```python
from build123d import *

# Parameters (mm, degrees)
BOSS_EXTRUDE1_DEPTH = 3.175
SKETCH2_R           = 1.5875
CUT_EXTRUDE1_DEPTH  = 3.175
BOSS_EXTRUDE2_DEPTH = 3.175
CUT_EXTRUDE2_DEPTH  = 3.175
SKETCH5_W           = 1.5875
SKETCH5_H           = 12.7
CUT_EXTRUDE3_DEPTH  = 10.16
LPATTERN1_COUNT     = 2
LPATTERN1_PITCH     = 25.4
SKETCH9_R           = 1.5875
CUT_EXTRUDE7_DEPTH  = 7.62
SKETCH10_R          = 6.35
CUT_EXTRUDE8_DEPTH  = 5.08


with BuildPart() as part:
    # Sketch1 → Boss-Extrude1 (new body)
    with BuildSketch(Plane.XY):
        Polygon((0, 0), (-177.8, 0), (-232.7656, 382.27), (-80.3656, 382.27), align=None)
    extrude(amount=BOSS_EXTRUDE1_DEPTH)

    # Sketch2 → Cut-Extrude1 (cut)
    with BuildSketch(Plane.XY.offset(3.175)):
        with Locations((-127, 127)):
            Circle(SKETCH2_R)
        with Locations((-127, 299.72)):
            Circle(SKETCH2_R)
    extrude(amount=-CUT_EXTRUDE1_DEPTH, mode=Mode.SUBTRACT)

    # Sketch3 → Boss-Extrude2 (add)
    with BuildSketch(Plane.XY.offset(3.175)):
        Polygon((-63.5, 82.55), (63.5, 104.94352655), (63.5, 181.14352655), (-63.5, 181.14352655), align=None)
    extrude(amount=-BOSS_EXTRUDE2_DEPTH)

    # Sketch4 → Cut-Extrude2 (cut)
    with BuildSketch(Plane.XY.offset(3.175)):
        Polygon((-57.15, 104.14), (-44.642941537, 106.345331856), (-45.194274501, 109.472096472), (-57.701332964, 107.266764616), align=None)
        Polygon((-19.62882461, 110.755995569), (-7.121766147, 112.961327425), (-7.673099111, 116.088092041), (-20.180157574, 113.882760185), align=None)
    extrude(amount=-CUT_EXTRUDE2_DEPTH, mode=Mode.SUBTRACT)

    # Sketch5 → Cut-Extrude3 (cut)
    with BuildSketch(Plane.XY.offset(3.175)):
        with Locations((-126.20625, 203.2)):
            Rectangle(SKETCH5_W, SKETCH5_H)
        with Locations((-127.79375, 203.2)):
            Rectangle(SKETCH5_W, SKETCH5_H)
    cut_extrude3 = extrude(amount=-CUT_EXTRUDE3_DEPTH, mode=Mode.SUBTRACT)

    # LPattern1: Cut-Extrude3 ×2
    with Locations(*[(0, i * LPATTERN1_PITCH, 0) for i in range(1, LPATTERN1_COUNT)]):
        add(cut_extrude3, mode=Mode.SUBTRACT)

    # Sketch9 → Cut-Extrude7 (cut)
    with BuildSketch(Plane(origin=(0, 0, 0), x_dir=(-1, 0, 0), z_dir=(0, 0, -1))):
        with Locations((171.45, 20.32)):
            Circle(SKETCH9_R)
        with Locations((44.45, 20.32)):
            Circle(SKETCH9_R)
    extrude(amount=-CUT_EXTRUDE7_DEPTH, mode=Mode.SUBTRACT)

    # Sketch10 → Cut-Extrude8 (cut)
    with BuildSketch(Plane(origin=(0, 0, 0), x_dir=(-1, 0, 0), z_dir=(0, 0, -1))):
        with Locations((156.845, 0)):
            Circle(SKETCH10_R)
        with Locations((66.04, 0)):
            Circle(SKETCH10_R)
    extrude(amount=-CUT_EXTRUDE8_DEPTH, mode=Mode.SUBTRACT)


solid = part.part
```
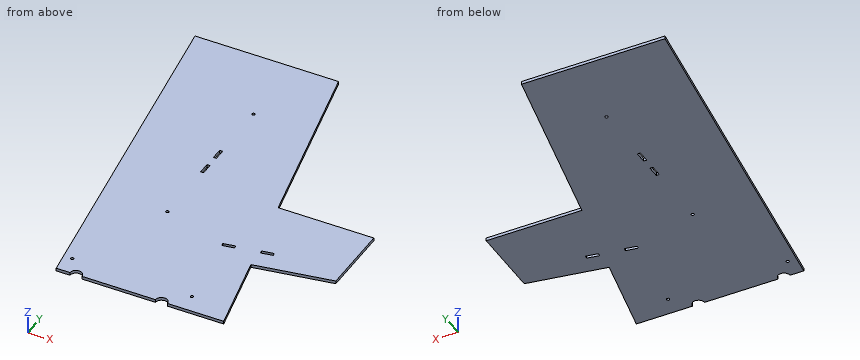
The model under review builds one solid part; all positions refer to its coordinate system, in mm. Round coordinates to 2 decimals unless told otherwise and drop trailing zeros. Loops run counter-clockwise (first coordinate to the right, second up) from the corner with the lowest first, then second, coordinate; pieces in that order, holes last.
1) Clearance check with flat-ended pins moving along their axes: P1, Ø1.6, axis at y = 202.5, z = 1, coming from the -X side; P2, Ø1.5, axis at y = 183.5, z = 2.5, coming from the -X side. State where each tip first meets the part, or that it passes through.
Values follow:
P1: stops at x = -207.03
P2: stops at x = -204.29
2) Consider section B-B on x = -66.04. State the section outline as (y, z) points (3 decimals), then the cut area to 3 significant figures.
Values follow:
outline: (6.35, 0) - (314.128, 0) - (314.128, 3.175) - (6.35, 3.175) - close
area: 977 mm2
3) Wall thickness on line 1 along Y through (x, z) = (-127, 2.15); line 2 along Y through (x, z) = (-171.45, 1.1); line 3 along Y through (x, z) = (-36, 0.95): over which ranges is each line inside the solid? List them lowest first.
Values follow:
line 1: y = 0 to 125.41, 128.59 to 196.85, 209.55 to 222.25, 234.95 to 298.13, 301.31 to 382.27
line 2: y = 0 to 18.73, 21.91 to 382.27
line 3: y = 0 to 181.14
4) Consider section A-A on z = 2.6. Give the number of separate pieces and of enclosed holes in the cut face, then the cut area to 3 significant figures.
Values follow:
separate pieces: 1
enclosed holes: 8
area: 70,500 mm2
